CAD build for the part. Positions are in the model's coordinates, mm. Face numbers are marked on the shaded views. A direction names the side the tool comes from. Coordinates: 2 decimals unless noted, no trailing zeros. Write each loop counter-clockwise with the first axis right and the second up, starting at its lowest first coordinate (ties: lowest second). Pieces come first, ordered by that corner, then holes. Notation, with made-up numbers: (23.25, 26.5) - (31.25, 26.5) arc R8 cw to (31.25, 40.5) - close; hole circle Ø4 at (82, 20). An arc over 180 degrees is marked (long way). Answer in a Markdown table with one row per item. Add a question column.
Q1. Band-saw the part on B-B (y = -13.25). State how many separate pieces and enclosed holes the cut face has, and give its area (3 significant figures).
Q2. Band-saw the part on D-D (x = 0). List the corners of the cut face in (y, z).
Q3. Drill centre lines: line 1 along X through (y, z) = (-8.5, 10); line 2 along Z through (x, y) = (-5.9, -18.75); line 3 along X through (y, z) = (-10.25, 12). Where is each one in solid material? Low to high. Write a range as from..to.
Q4. Band-saw the part on A-A (x = -25). List the corners of the cut face in (y, z).
Q5. Band-saw the part on C-C (z = 2.5). List the corners of the cut face in (x, y).
Q6. Pin check, flat tips, straight feed: pin 1 (4 mm diameter, centred on y = -14, z = 10, fed in from -X); pin 2 (1.9 mm diameter, centred on x = 24.5, y = -13.5, fed in from +Z); pin 3 (1 mm diameter, centred on y = -17, z = 2, fed in from -X). Stop position of each tip, or through.
Q7. 3-axis set-ups, long thin cutter, end or side, ignore diameter. For the marked faces 1, 2 and 3: which of +Z, -Z, +X, -X, +Y, -Y reach the whole face in a straight line?
Q8. Two-plate mould, pull along X, no slides. Class the marked faces 4, 5 and 6: +X half, -X half, draft (parallel to the pull), parting line (faces both ways), or undercut.
```python
from build123d import *

# Parameters (mm, degrees)
F1_DEPTH  = 25
F2_R      = 1.55
F3_DEPTH  = 25
F4_R      = 1.5
F5_DEPTH  = 25
F6_R      = 3.3134143982
F9_DEPTH  = 1.2
F8_R      = 1.5
F10_DEPTH = 1.2
F12_DEPTH = 1.2
F13_R     = 0.5


# Not quite as in the source:
# - ends of sketch curves that miss each other by under 0.0002 mm in the source are joined


with BuildPart() as f1:
    # F0 (on Front) → F1 (new body)
    with BuildSketch(Plane.XZ):
        with BuildLine():
            Line((-30, -26.7712218283), (30, -26.771222222))
            Line((30, -26.771222222), (30, -22.771222222))
            Line((30, -22.771222222), (11.8647393899, -22.7712218283))
            ThreePointArc((11.8647393899, -22.7712218283), (16.8306466966, -8.2027211962), (8, 4.4036710302))
            Line((8, 4.4036710302), (8, 14.4036710302))
            Line((8, 14.4036710302), (3, 14.4036710302))
            Line((3, 14.4036710302), (3, 6.1368714524))
            Line((3, 6.1368714524), (3, 4.8868714524))
            Line((3, 4.8868714524), (3, 1.0226200218))
            ThreePointArc((3, 1.0226200218), (0, -22.5963300169), (-3, 1.0226200218))
            Line((-3, 1.0226200218), (-3, 4.8868714524))
            Line((-3, 4.8868714524), (-3, 14.4036710302))
            Line((-3, 14.4036710302), (-8, 14.4036710302))
            Line((-8, 14.4036710302), (-8, 4.4036710302))
            ThreePointArc((-8, 4.4036710302), (-16.8306466966, -8.2027211962), (-11.8647393899, -22.7712218283))
            Line((-11.8647393899, -22.7712218283), (-30, -22.7712218283))
            Line((-30, -22.7712218283), (-30, -26.7712218283))
        make_face()
    extrude(amount=F1_DEPTH)

    # F2 (on face) → F3 (cut)
    with BuildSketch(Plane.XY.offset(-22.7712218283)):
        with Locations((-25, -12.5)):
            Circle(F2_R)
        with Locations((25, -12.5)):
            Circle(F2_R)
    extrude(amount=-F3_DEPTH, mode=Mode.SUBTRACT)

    # F4 (on face) → F5 (cut)
    with BuildSketch(Plane.YZ.offset(8)):
        with Locations((-18.75, 9.4036710302)):
            Circle(F4_R)
        with Locations((-6.25, 9.4036710302)):
            Circle(F4_R)
    extrude(amount=-F5_DEPTH, mode=Mode.SUBTRACT)

    # F6
    f6_edges = [f1.edges().sort_by_distance(p)[0] for p in [
        (-5.5, -25, 14.403671),
        (5.5, -25, 14.403671),
        (-5.5, 0, 14.403671),
        (5.5, 0, 14.403671),
        (30, -25, -24.771222),
        (30, 0, -24.771222),
        (-30, 0, -24.771222),
        (-30, -25, -24.771222),
        (11.864739, -12.5, -22.771222),
        (-11.864739, -12.5, -22.771222),
    ]]
    fillet(f6_edges, radius=F6_R)

    # F7 (on face) → F9 (cut)
    with BuildSketch(Plane.YZ.offset(8)):
        Polygon((-20.55, 6.2859795766), (-16.95, 6.2859795766), (-15.15, 9.4036710302), (-16.95, 12.5213624838), (-20.55, 12.5213624838), (-22.35, 9.4036710302), align=None)
        Polygon((-4.45, 12.5213624838), (-8.05, 12.5213624838), (-9.85, 9.4036710302), (-8.05, 6.2859795766), (-4.45, 6.2859795766), (-2.65, 9.4036710302), align=None)
    extrude(amount=-F9_DEPTH, mode=Mode.SUBTRACT)

    # F8 (on face) → F10 (cut)
    with BuildSketch(Plane(origin=(-8, 0, 0), x_dir=(0, -1, 0), z_dir=(-1, 0, 0))):
        Polygon((4.45, 6.2859795766), (8.05, 6.2859795766), (9.85, 9.4036710302), (8.05, 12.5213624838), (4.45, 12.5213624838), (2.65, 9.4036710302), align=None)
        with Locations((6.25, 9.4036710302)):
            Circle(F8_R, mode=Mode.SUBTRACT)
        Polygon((20.55, 12.5213624838), (16.95, 12.5213624838), (15.15, 9.4036710302), (16.95, 6.2859795766), (20.55, 6.2859795766), (22.35, 9.4036710302), align=None)
        with Locations((18.75, 9.4036710302)):
            Circle(F8_R, mode=Mode.SUBTRACT)
    extrude(amount=-F10_DEPTH, mode=Mode.SUBTRACT)

    # F11 (on face) → F12 (cut)
    with BuildSketch(Plane.XY.offset(-22.7712218283)):
        Polygon((26.8, -9.3823085464), (23.2, -9.3823085464), (21.4, -12.5), (23.2, -15.6176914536), (26.8, -15.6176914536), (28.6, -12.5), align=None)
        Polygon((-23.2, -15.6176914536), (-21.4, -12.5), (-23.2, -9.3823085464), (-26.8, -9.3823085464), (-28.6, -12.5), (-26.8, -15.6176914536), align=None)
    extrude(amount=-F12_DEPTH, mode=Mode.SUBTRACT)

    # F13
    f13_edges = [f1.edges().sort_by_distance(p)[0] for p in [
        (0, 0, -22.59633),
        (0, -25, -22.59633),
    ]]
    fillet(f13_edges, radius=F13_R)


solid = f1.part
```
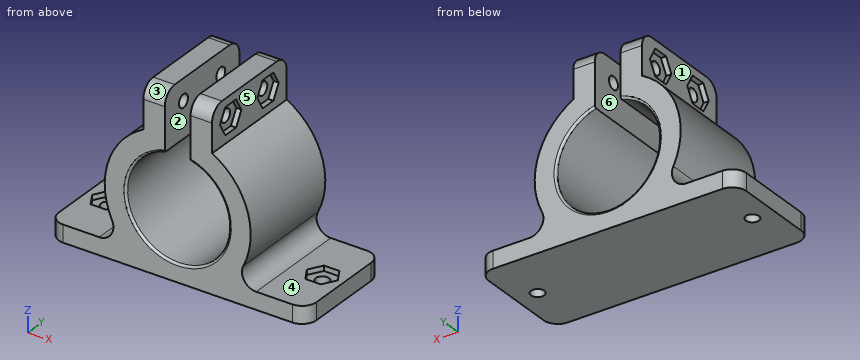
Checked values:
| question | item | result |
|---|---|---|
| 1 | separate pieces | 3 |
| 1 | enclosed holes | 0 |
| 1 | area | 662 mm² |
| 2 | outline | (-25, -26.77) - (0, -26.77) - (0, -23.1) arc R0.5 ccw to (-0.5, -22.6) - (-24.5, -22.6) arc R0.5 ccw to (-25, -23.1) - close |
| 3 | line 1 | x = -6.8..-3, 3..6.8 |
| 3 | line 2 | z = -26.77..-21.05, -0.15..7.9, 10.9..14.4 |
| 3 | line 3 | x = -8..-3, 3..8 |
| 4 | outline | (-25, -26.77) - (-14.05, -26.77) - (-14.05, -23.97) - (-15.62, -23.97) - (-15.62, -22.77) - (-25, -22.77) - close; (-10.95, -26.77) - (0, -26.77) - (0, -22.77) - (-9.38, -22.77) - (-9.38, -23.97) - (-10.95, -23.97) - close |
| 5 | outline | (-10.84, -25) - (-3, -25) - (-3, 0) - (-10.84, 0) - close; (3, -25) - (10.84, -25) - (10.84, 0) - (3, 0) - close |
| 6 | pin 1 | stops at x = -8 |
| 6 | pin 2 | stops at z = -23.97 |
| 6 | pin 3 | stops at x = -11.94 |
| 7 | face 1 | +Z, -X, +Y, -Y |
| 7 | face 2 | +Z, +Y, -Y |
| 7 | face 3 | +Z, +X, -X, -Y |
| 8 | face 4 | draft |
| 8 | face 5 | +X half |
| 8 | face 6 | undercut |
